```python
from build123d import *

# Parameters (mm, degrees)
F0_R     = 31.75
F0_R_2   = 3.175
F0_R_3   = 12.7
F1_DEPTH = 2.54


with BuildPart() as f1:
    # F0 (on Front) → F1 (new body)
    with BuildSketch(Plane.XZ):
        Circle(F0_R)
        with Locations((-8.89, -15.397932)):
            Circle(F0_R_2, mode=Mode.SUBTRACT)
        with Locations((8.89, -15.397932)):
            Circle(F0_R_2, mode=Mode.SUBTRACT)
        with Locations((-17.78, 0)):
            Circle(F0_R_2, mode=Mode.SUBTRACT)
        with Locations((-8.89, 15.397932)):
            Circle(F0_R_2, mode=Mode.SUBTRACT)
        Circle(F0_R_3, mode=Mode.SUBTRACT)
        with Locations((8.89, 15.397932)):
            Circle(F0_R_2, mode=Mode.SUBTRACT)
        with Locations((17.78, 0)):
            Circle(F0_R_2, mode=Mode.SUBTRACT)
    extrude(amount=F1_DEPTH)


solid = f1.part
```
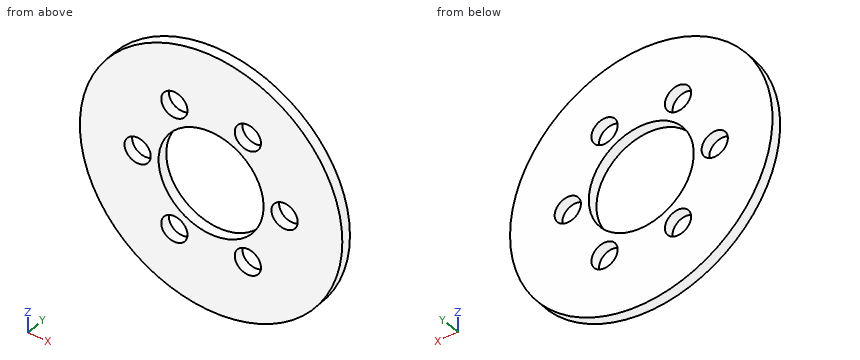
Source: CAD feature listing. Evaluate the final solid. Frame: model axes, mm. Coordinates: 2 decimals unless noted, no trailing zeros. Loops run counter-clockwise (first coordinate to the right, second up) from the corner with the lowest first, then second, coordinate; pieces in that order, holes last. Notation, with made-up numbers: (0, 60.5) -> (33, 60.5) arc R19 ccw to (33, 93.5) -> close; hole circle Ø10 at (-31.5, -11). An arc over 180 degrees is marked (long way). One line per item, written item: value. Start each with the question number.
Q1. Line query: line 1 along Z through (x, y) = (-8.89, -1.3); line 2 along Z through (x, y) = (0, -1.6); line 3 along Z through (x, y) = (-11, -0.2). Output: solid intervals per line, ascending.
Q2. Section query C-C, the plane y = -1.4. Return the cut outline in (x, z) (3 decimals), and give its area (3 significant figures).
Q3. Contact query for flat-ended pins moving along their axis: P1, Ø10, axis at x = 8.89, z = 15.4, coming from the -Y side; P2, Ø1, axis at y = -2, z = 13.5, coming from the -X side. Output: stop coordinate, or through.
Q4. Section query B-B, the plane z = 0. Return the cut outline in (x, y) (3 decimals), and give its area (3 significant figures).
Q5. Section query A-A, the plane x = 0. Return the cut outline in (y, z).
Q6. Section query D-D, the plane z = -9. Return the cut outline in (x, y).
Results:
1. line 1: -30.48 to -18.57, -12.22 to -9.07, 9.07 to 12.22, 18.57 to 30.48
1. line 2: -31.75 to -12.7, 12.7 to 31.75
1. line 3: -29.78 to -17.77, -13.03 to -6.35, 6.35 to 13.03, 17.77 to 29.78
2. outline: circle Ø63.5 at (0, 0); hole circle Ø6.35 at (-17.78, 0); hole circle Ø25.4 at (0, 0); hole circle Ø6.35 at (-8.89, -15.398); hole circle Ø6.35 at (-8.89, 15.398); hole circle Ø6.35 at (8.89, -15.398); hole circle Ø6.35 at (8.89, 15.398); hole circle Ø6.35 at (17.78, 0)
2. area: 2,470 mm^2
3. P1: y = -2.54
3. P2: x = -28.97
4. outline: (-31.75, -2.54) -> (-20.955, -2.54) -> (-20.955, 0) -> (-31.75, 0) -> close; (-14.605, -2.54) -> (-12.7, -2.54) -> (-12.7, 0) -> (-14.605, 0) -> close; (12.7, -2.54) -> (14.605, -2.54) -> (14.605, 0) -> (12.7, 0) -> close; (20.955, -2.54) -> (31.75, -2.54) -> (31.75, 0) -> (20.955, 0) -> close
4. area: 64.5 mm^2
5. outline: (-2.54, -31.75) -> (0, -31.75) -> (0, -12.7) -> (-2.54, -12.7) -> close; (-2.54, 12.7) -> (0, 12.7) -> (0, 31.75) -> (-2.54, 31.75) -> close
6. outline: (-30.45, -2.54) -> (-8.96, -2.54) -> (-8.96, 0) -> (-30.45, 0) -> close; (8.96, -2.54) -> (30.45, -2.54) -> (30.45, 0) -> (8.96, 0) -> close
